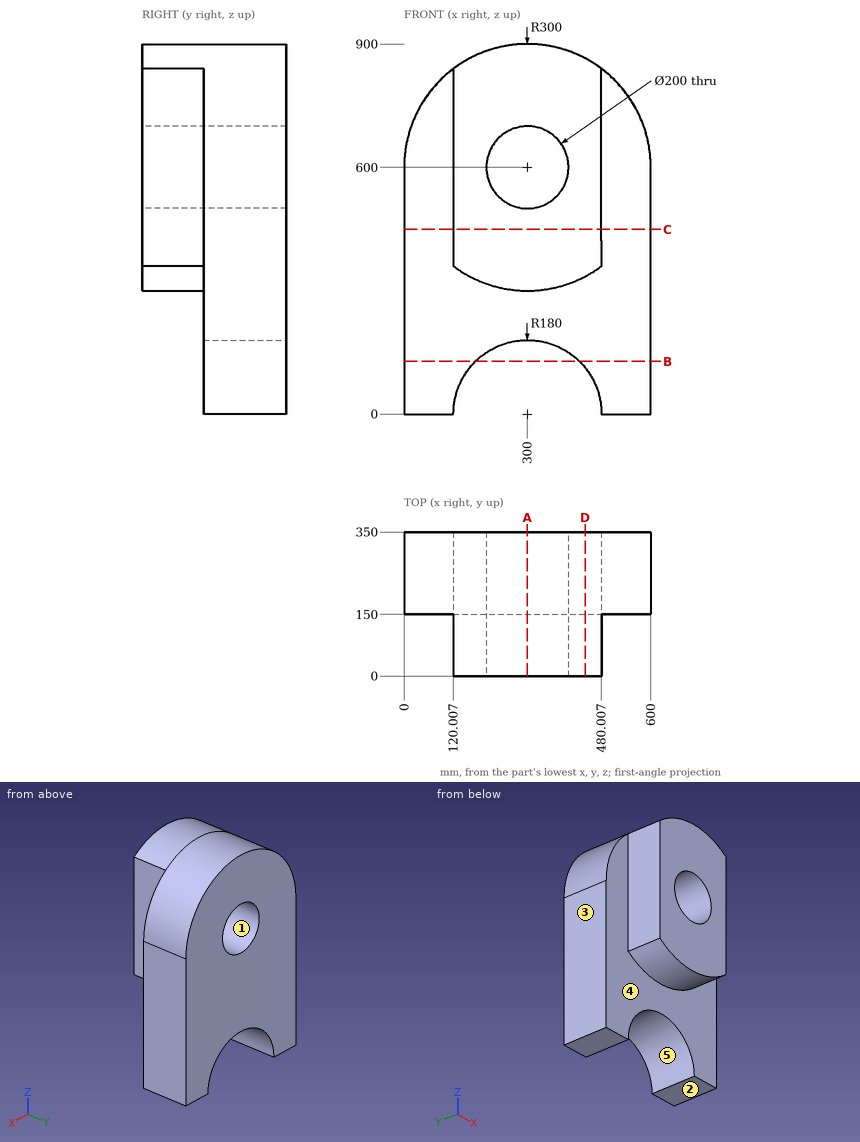
Can you work these out from the drawing? Everything is in mm from the part's minimum corner. A direction names the side the tool comes from. Give positions to 0.01 mm unless a question says otherwise; leave off trailing zeros. Order: outer loops, then holes, each group sorted by start corner. A loop starts at its lowest first (then second) coordinate and runs counter-clockwise, first axis right, second up.
Item 1: I'm going to push flat-ended pins straight in: pin 1 (4 mm diameter, centred on y = 274, z = 668, fed in from -X); pin 2 (10 mm diameter, centred on x = 213.5, y = 108, fed in from -Z); pin 3 (4 mm diameter, centred on x = 128, y = 293.5, fed in from +Z) (1 decimal). Where does each tip first touch, or does it pass through?
Item 2: If we section it at D-D, the plane x = 440.5: Write out the boundary of the cut face in (y, z) (1 decimal).
Item 3: If we mould it in two halves opening along X, with no side actions, what happens to the marked faces 1, 2 and 3? For each: pulls with the +X half, pulls with the -X half, needs draft (parallel to the pull), parting line crosses it, or undercut.
Item 4: For the marked faces 4 and 5, which set-ups out of +Z, -Z, +X, -X, +Y, -Y let a thin tool reach every point of the face, with its end or its side?
Item 5: If we section it at C-C, the plane z = 449: Write out the boundary of the cut face in (x, y) (1 decimal).
Item 6: If we section it at A-A, the plane x = 300: Write out the boundary of the cut face in (y, z), plus the area to 3 significant figures.
Item 7: I need wall thicknesses on line 1 (Z direction, x = 300, y = 215); line 2 (Z direction, x = 300, y = 125); line 3 (Y direction, x = 321.5, z = 288.5). Which ranges of each line are inside material? Lowest first, please.
Item 8: If we section it at B-B, the plane z = 128: Write out the boundary of the cut face in (x, y).
Values:
1. pin 1: stops at x = 7.35
1. pin 2: stops at z = 311.28
1. pin 3: stops at z = 847.2
2. outline: (0, 334.9) - (150, 334.9) - (150, 112.5) - (350, 112.5) - (350, 865.1) - (0, 865.1) - close
3. face 1: undercut
3. face 2: needs draft
3. face 3: pulls with the -X half
4. face 4: -Z, -Y
4. face 5: -Z, +Y, -Y
5. outline: (0, 150) - (120.1, 150) - (120.1, 0) - (480.1, 0) - (480.1, 150) - (600, 150) - (600, 350) - (0, 350) - close
6. outline: (0, 300) - (150, 300) - (150, 180) - (350, 180) - (350, 500) - (0, 500) - close; (0, 700) - (350, 700) - (350, 900) - (0, 900) - close
6. area: 164,000 mm2
7. line 1: z = 180 to 500, 700 to 900
7. line 2: z = 300 to 500, 700 to 900
7. line 3: y = 150 to 350
8. outline: (0, 150) - (173.45, 150) - (173.45, 350) - (0, 350) - close; (426.55, 150) - (600, 150) - (600, 350) - (426.55, 350) - close
